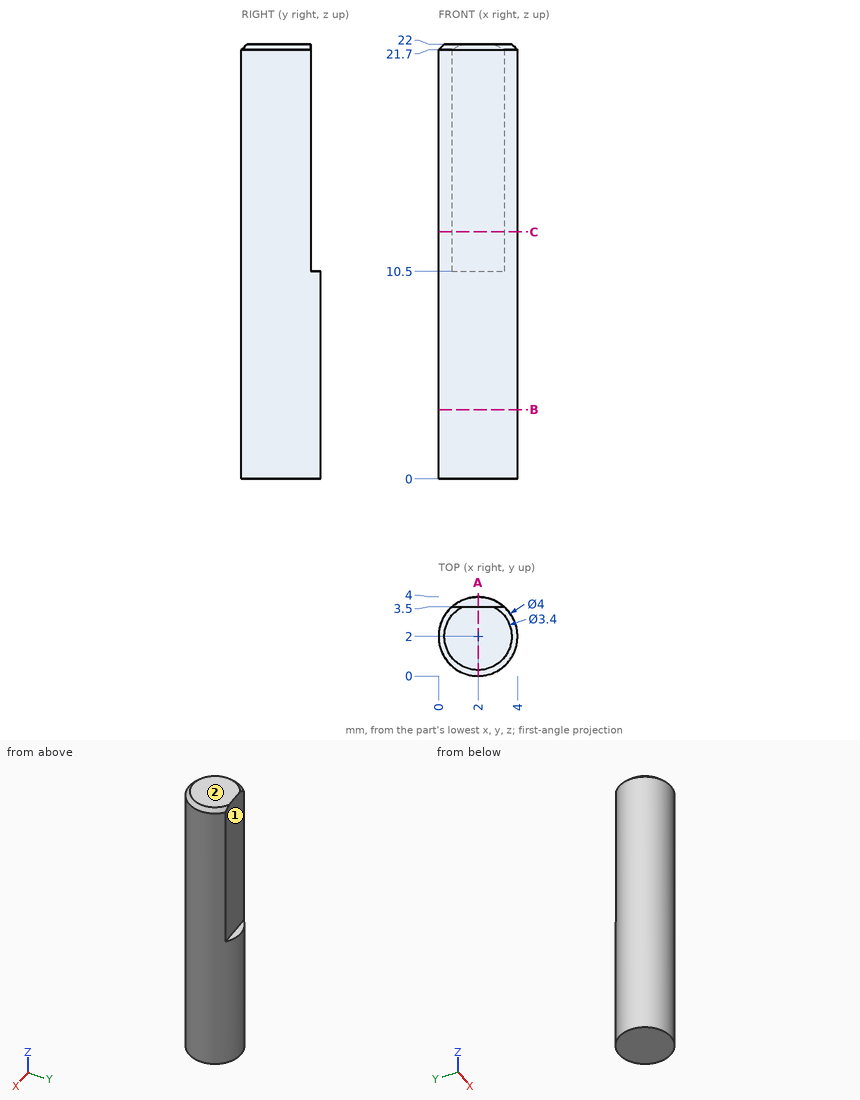
Design review of the part shown in the three views and the two pictorial views. Dimensions are in mm from the part's minimum x, y and z. A direction names the side the tool comes from. Coordinates: 2 decimals unless noted, no trailing zeros. Write each loop counter-clockwise with the first axis right and the second up, starting at its lowest first coordinate (ties: lowest second). Pieces come first, ordered by that corner, then holes.
1) We need section B-B on z = 3.5. State the section outline as (x, y) points.
2) We need section C-C on z = 12.5. State the section outline as (x, y) points.
3) To check wall thickness, follow probe 1 along Y at (x, z) = (2.05, 14); probe 2 along Y at (x, z) = (3.5, 6.75); probe 3 along X at (y, z) = (1, 17). State the ranges of each line that lie inside material, in increasing order.
4) Machinability: for the marked faces 1 and 2, which of the approach directions +Z, -Z, +X, -X, +Y, -Y give a long, thin tool a straight path to every point of the face, cutting with its end or side? Answer none if there is none.
5) Clearance check with flat-ended pins moving along their axes: pin 1 Ø1.3 at (x, z) = (2, 19) entering from +Y; pin 2 Ø1.5 at (y, z) = (1, 9) entering from -X. State where each tip first meets the part, or that it passes through.
6) We need section A-A on x = 2. State the section outline as (y, z) points, then the cut area to 3 significant figures.
Answer list:
1. outline: circle Ø4 at (2, 2)
2. outline: (0.68, 3.5) arc R2 ccw (long way) to (3.32, 3.5) - close
3. probe 1: y = 0 to 3.5
3. probe 2: y = 0.68 to 3.32
3. probe 3: x = 0.27 to 3.73
4. face 1: +Z, +X, -X, +Y
4. face 2: +Z, +X, -X, +Y, -Y
5. pin 1: stops at y = 3.5
5. pin 2: stops at x = 0.02
6. outline: (0, 0) - (4, 0) - (4, 10.5) - (3.5, 10.5) - (3.5, 22) - (0.3, 22) - (0, 21.7) - close
6. area: 82.2 mm2
